For this review, take the finished solid that the model builds, in its own axes (mm). Round coordinates to 2 decimals unless told otherwise and drop trailing zeros. Loops run counter-clockwise (first coordinate to the right, second up) from the corner with the lowest first, then second, coordinate; pieces in that order, holes last.
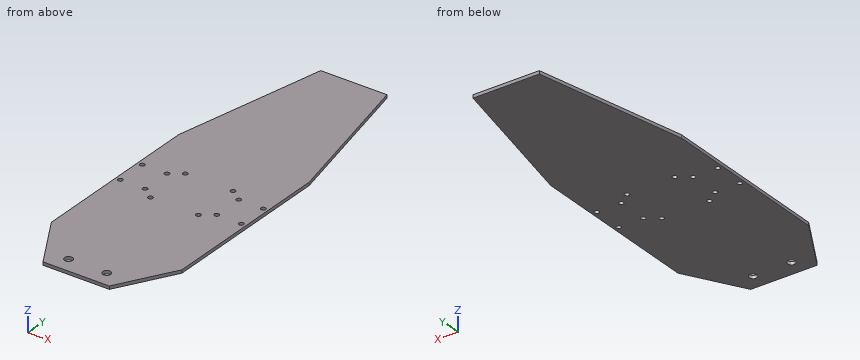
```python
from build123d import *

# Parameters (mm, degrees)
F0_W     = 82
F0_H     = 110
F1_DEPTH = 2
F3_D     = 3
F5_D     = 5
F7_D     = 3


with BuildPart() as f1:
    # F0 (on Top) → F1 (new body)
    with BuildSketch(Plane.XY):
        Polygon((20.1851744205, 205), (0, 110), (82, 110), (61.8148255795, 205), align=None)
        with Locations((41, 55)):
            Rectangle(F0_W, F0_H)
        Polygon((82, 0), (0, 0), (20.1851744205, -35), (61.8148255795, -35), align=None)
    extrude(amount=F1_DEPTH)

    # F3 (through all)
    with Locations(Plane.XY.offset(2)):
        with Locations((18.5, 55.5), (3, 55.5), (3, 74.5), (18.5, 74.5), (63.5, 74.5), (63.5, 55.5), (79, 55.5), (79, 74.5)):
            Hole(F3_D / 2)

    # F5 (through all)
    with Locations(Plane.XY.offset(2)):
        with Locations((29, -25), (53, -25)):
            Hole(F5_D / 2)

    # F7 (through all)
    with Locations(Plane.XY.offset(2)):
        with Locations((26, 80), (56, 50), (56, 80), (26, 50)):
            Hole(F7_D / 2)


solid = f1.part
```
(1) Add section A-A (z = 0.7). Give the number of separate pieces and of enclosed holes in the cut face, plus the area to 3 significant figures.
(2) For L1, parallel to X at y = 74.5, z = 1.65; L2, parallel to Y at x = 26, z = 1.2; L3, parallel to X at y = 192.5, z = 1.4, list the stretches that pass through material, from the lowest coordinate up.
(3) Add section C-C (x = 12). Give the boundary of the cut face in (y, z).
(4) Add section B-B (y = -25). Give the boundary of the cut face in (x, z).
(5) Add section D-D (y = 188). Give the boundary of the cut face in (x, z).
Outcome:
1. separate pieces: 1
1. enclosed holes: 14
1. area: 16,900 mm2
2. L1: x = 0 to 1.5, 4.5 to 17, 20 to 62, 65 to 77.5, 80.5 to 82
2. L2: y = -35 to 48.5, 51.5 to 78.5, 81.5 to 205
2. L3: x = 17.53 to 64.47
3. outline: (-20.81, 0) - (166.48, 0) - (166.48, 2) - (-20.81, 2) - close
4. outline: (14.42, 0) - (26.5, 0) - (26.5, 2) - (14.42, 2) - close; (31.5, 0) - (50.5, 0) - (50.5, 2) - (31.5, 2) - close; (55.5, 0) - (67.58, 0) - (67.58, 2) - (55.5, 2) - close
5. outline: (16.57, 0) - (65.43, 0) - (65.43, 2) - (16.57, 2) - close
